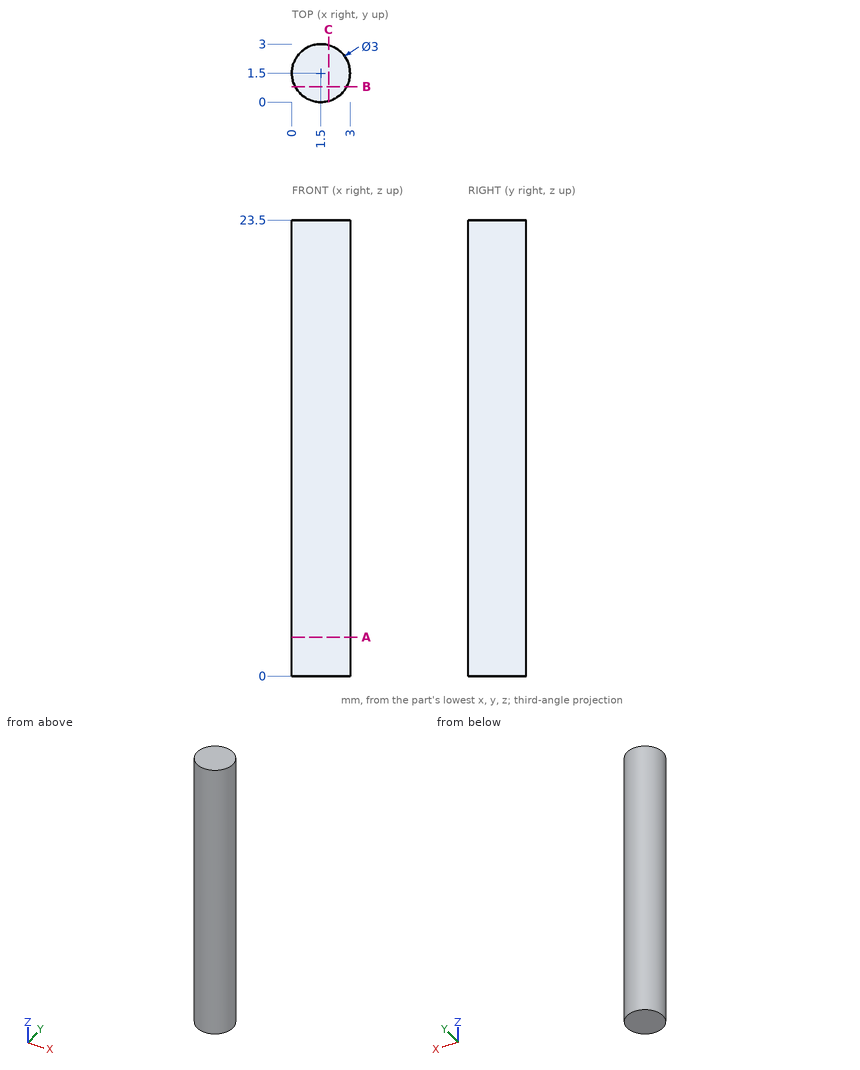
Here's the drawing with two shaded views (mm, measured from the low corner). I have some questions. Give positions to 0.01 mm unless a question says otherwise; leave off trailing zeros. Order: outer loops, then holes, each group sorted by start corner. A loop starts at its lowest first (then second) coordinate and runs counter-clockwise, first axis right, second up. Notation, with made-up numbers: (14, 74) - (65, 74) arc R26 cw to (65, 113) - close; hole circle Ø3 at (-37.5, 37.25). An arc over 180 degrees is marked (long way). Use a Markdown table: item, result. Add a question column.
Q1. If we section it at B-B on y = 0.8: Write out the boundary of the cut face in (x, z).
Q2. Please list where these lines run through material, in increasing order: line 1 along Y through (x, z) = (2, 11.5); line 2 along X through (y, z) = (1.4, 6.75); line 3 along X through (y, z) = (0.85, 2.25).
Q3. If we section it at A-A on z = 2: Write out the boundary of the cut face in (x, y), plus the area to 3 significant figures.
Q4. If we section it at C-C on x = 1.9: Write out the boundary of the cut face in (y, z).
Answers follow:
| question | item | result |
|---|---|---|
| 1 | outline | (0.17, 0) - (2.83, 0) - (2.83, 23.5) - (0.17, 23.5) - close |
| 2 | line 1 | y = 0.09 to 2.91 |
| 2 | line 2 | x = 0 to 3 |
| 2 | line 3 | x = 0.15 to 2.85 |
| 3 | outline | circle Ø3 at (1.5, 1.5) |
| 3 | area | 7.07 mm^2 |
| 4 | outline | (0.05, 0) - (2.95, 0) - (2.95, 23.5) - (0.05, 23.5) - close |
